Could you check a few things on this model? Use its own coordinates, in mm. Give positions to 0.01 mm unless a question says otherwise; leave off trailing zeros. Loops run counter-clockwise (first coordinate to the right, second up) from the corner with the lowest first, then second, coordinate; pieces in that order, holes last.
1. Imagine slicing it at A-A (x = 6.25). List the corners of the cut face in (y, z) for me (3 decimals), plus the area to 3 significant figures.
2. I need wall thicknesses on line 1 along Z through (x, y) = (6.25, 0.55); line 2 along X through (y, z) = (-0.45, 0); line 3 along Z through (x, y) = (5.5, 2.6). Which ranges of each line are inside material? Lowest first, please.
3. Thinking about a two-plate mould opening in X: for faces 1 (the flat face through (3, 2.875, 0)), 2 (the cylindrical face through (5.06, 0.04, 0.91)), 3 (the flat face through (-6.25, 0, 0)), 4 (the flat face through (18.718, 0, 0)), which applies, +X half, -X half, draft (parallel to the pull), parting line (faces both ways), or undercut?
4. Imagine slicing it at B-B (z = 0). List the corners of the cut face in (x, y) for me (3 decimals), plus the area to 3 significant figures.
Autodesk Inventor part; units mm, degrees
ref_plane "YZ Plane" through (0, 0, 0) normal (1, 0, 0) x (0, 1, 0)
ref_plane "XZ Plane" through (0, 0, 0) normal (0, 1, 0) x (-1, 0, 0)
ref_plane "XY Plane" through (0, 0, 0) normal (0, 0, 1) x (1, 0, 0)
sketch "Sketch1" plane through (0, 0, 0) normal (1, 0, 0) x (0, 1, 0)
  line L0 (2.875, -19) -> (-2.875, -19)
  line L1 (-2.875, -19) -> (-2.875, 19)
  line L2 (-2.875, 19) -> (2.875, 19)
  line L3 (2.875, 19) -> (2.875, -19)
  line L4 (2.875, -19) -> (-2.875, 19) construction
  line L5 (-2.875, -19) -> (2.875, 19) construction
  point P0 (0, 0)
  dimension "d0" = 5.75
  dimension "d1" = 38
extrude "Extrusion1" add sketch "Sketch1" along normal blind 12.5
sketch "Sketch2" plane through (0, 2.875, 19) normal (0, 1, 0) x (1, 0, 0)
  circle A0 centre (6.25, 19) radius 1.5
  point P0 (0, 19)
  dimension "d4" = 3
extrude "Extrusion2" cut sketch "Sketch2" against normal blind 12.5
sketch "Sketch3" plane through (12.5, 0, 0) normal (1, 0, 0) x (0, 0, -1)
  point P0 (0, 0)
sketch "Sketch4" plane through (0, -2.875, -19) normal (0, -1, 0) x (1, 0, 0)
  line L0 (0, 0) -> (0, 38)
  line L1 (0, 0) -> (-6.25, 0)
  line L2 (-6.25, 0) -> (-6.25, 38)
  line L3 (-6.25, 38) -> (0, 38)
  line L4 (0, 38) -> (0, 0)
  line L5 (12.4682, 38) -> (18.7182, 38)
  line L6 (18.7182, 38) -> (18.7182, 0)
  line L7 (18.7182, 0) -> (12.4682, 0)
  line L8 (12.4682, 0) -> (12.4682, 38)
  point P0 (0, 19)
  dimension "d7" = 6.25
  dimension "d8" = 6.25
extrude "Extrusion3" add sketch "Sketch4" against normal up to surface (5.75 mm away)
properties part number "servoArm"
Derived:
1. outline: (-2.875, -19) - (2.875, -19) - (2.875, -1.5) - (-2.875, -1.5) - close; (-2.875, 1.5) - (2.875, 1.5) - (2.875, 19) - (-2.875, 19) - close
1. area: 201 mm2
2. line 1: z = -19 to -1.5, 1.5 to 19
2. line 2: x = -6.25 to 4.75, 7.75 to 18.72
2. line 3: z = -19 to -1.3, 1.3 to 19
3. face 1: draft
3. face 2: undercut
3. face 3: -X half
3. face 4: +X half
4. outline: (-6.25, -2.875) - (4.75, -2.875) - (4.75, 2.875) - (-6.25, 2.875) - close; (7.75, -2.875) - (18.718, -2.875) - (18.718, 2.875) - (7.75, 2.875) - close
4. area: 126 mm2
